Geometry: final body of the model. Coordinates: model frame, mm. A direction names the side the tool comes from. Give positions to 0.01 mm unless a question says otherwise; leave off trailing zeros. Order: outer loops, then holes, each group sorted by start corner. A loop starts at its lowest first (then second) coordinate and runs counter-clockwise, first axis right, second up. Notation, with made-up numbers: (83.5, -12) - (123.5, -12) arc R26 cw to (123.5, 8) - close; hole circle Ø3 at (51.25, 27). An arc over 180 degrees is marked (long way). One line per item, written item: value.
```python
from build123d import *

# Parameters (mm, degrees)
CIRCULARBAND_W               = 50
CIRCULARBAND_H               = 2.5
BASE_REVOLVE_ANGLE           = 120
BASE_REVOLVE_OTHER_WAY_ANGLE = 120
SKETCH9_OUTSIDE_W            = 80.09
SKETCH9_OUTSIDE_H            = 108.84
HEAD1_DEPTH                  = 53.5
SKETCH10_OUTSIDE_W           = 80.09
SKETCH10_OUTSIDE_H           = 108.84
TAIL1_DEPTH                  = 53.5


with BuildPart() as part:
    # circularband → Base-Revolve (revolve)
    with BuildSketch(Plane.XY):
        with Locations((0, 51.25)):
            Rectangle(CIRCULARBAND_W, CIRCULARBAND_H)
    revolve(axis=Axis((0, 0, 0), (1, 0, 0)), revolution_arc=BASE_REVOLVE_ANGLE)

    # circularband → Base-Revolve other way (revolve)
    with BuildSketch(Plane.XY):
        with Locations((0, 51.25)):
            Rectangle(CIRCULARBAND_W, CIRCULARBAND_H)
    revolve(axis=Axis((0, 0, 0), (-1, 0, 0)), revolution_arc=BASE_REVOLVE_OTHER_WAY_ANGLE)

    # Sketch9 outside → head1 (cut, through all)
    with BuildSketch(Plane.XY):
        with Locations((0, 13.125)):
            Rectangle(SKETCH9_OUTSIDE_W, SKETCH9_OUTSIDE_H)
        Polygon((-11.25, 52.5), (11.25, 52.5), (11.25, 19.301270189), (25, 19.301270189), (0, -24), (-25, 19.301270189), (-11.25, 19.301270189), align=None, mode=Mode.SUBTRACT)
    extrude(amount=-HEAD1_DEPTH, mode=Mode.SUBTRACT)

    # Sketch10 outside → tail1 (cut, through all)
    with BuildSketch(Plane.XY):
        with Locations((0, 13.125)):
            Rectangle(SKETCH10_OUTSIDE_W, SKETCH10_OUTSIDE_H)
        Polygon((0, -6.764428415), (11.25, -26.25), (11.25, 52.5), (-11.25, 52.5), (-11.25, -26.25), align=None, mode=Mode.SUBTRACT)
    extrude(amount=TAIL1_DEPTH, mode=Mode.SUBTRACT)


solid = part.part
```
1) First-contact query: pin 1 (1.5 mm diameter, centred on x = 8.5, y = 29, fed in from -Z); pin 2 (0.8 mm diameter, centred on x = 15.5, z = -48, fed in from +Y); pin 3 (3 mm diameter, centred on x = 18, y = 20, fed in from -Z). Flat tips, straight axial feed; report the tip coordinate or a pass-through.
Answers below:
pin 1: z = -44.25
pin 2: y = 19.3
pin 3: z = -49.13
2) Section A-A, the plane y = 8. Return loops of the section in (x, z), then the cut area to 3 significant figures.
Answers below:
outline: (-18.48, -51.89) - (18.48, -51.89) - (18.48, -49.36) - (-18.48, -49.36) - close; (-11.25, 49.36) - (11.25, 49.36) - (11.25, 51.89) - (-11.25, 51.89) - close
area: 150 mm^2
3) Mould query, pull axis Z, two halves, no side actions, for faces 4 (the face through (0.35, 52.425, 2.802)), 5 (the face through (0.35, 45.61, -20.49)), 6 (the face through (18, 19.301, -47)). Classes: released by +Z, released by -Z, zero draft, split by the parting line, or undercut.
Answers below:
face 4: split by the parting line
face 5: undercut
face 6: zero draft
4) Section C-C, the plane z = 0. Return loops of the section in (x, y).
Answers below:
outline: (-11.25, 50) - (11.25, 50) - (11.25, 52.5) - (-11.25, 52.5) - close
5) Material intervals for line 1 along Z through (x, y) = (-1, 0); line 2 along Y through (x, z) = (-4, 0); line 3 along Z through (x, y) = (2.5, 6), sorted ascending.
Answers below:
line 1: -52.5 to -50, 50 to 52.5
line 2: 50 to 52.5
line 3: -52.16 to -49.64, 49.64 to 52.16
6) Section B-B, the plane y = -9. Return loops of the section in (x, z), then the cut area to 3 significant figures.
Answers below:
outline: (-11.25, 49.18) - (-1.29, 49.18) - (-1.29, 51.72) - (-11.25, 51.72) - close; (-8.66, -51.72) - (8.66, -51.72) - (8.66, -49.18) - (-8.66, -49.18) - close; (1.29, 49.18) - (11.25, 49.18) - (11.25, 51.72) - (1.29, 51.72) - close
area: 94.6 mm^2
7) Set-up query: faces 1 (the face through (12.558, -2.248, -50.721)), 2 (the face through (-18, 19.301, -47)), 3 (the face through (-12.44, -2.45, -50.4)). Return all of +Z, -Z, +X, -X, +Y, -Y with unobstructed straight access to the full face (end or side cutting, diameter ignored); none if empty.
Answers below:
face 1: -Z, +X, -Y
face 2: +Z, -Z, -X, +Y
face 3: -Z, -X, -Y
8) Section D-D, the plane x = 2.5. Return loops of the section in (y, z), then the cut area to 3 significant figures.
Answers below:
outline: (-19.67, -48.68) arc R52.5 ccw (long way) to (-11.09, 51.31) - (-11.09, 48.75) arc R50 cw (long way) to (-19.67, -45.97) - close
area: 481 mm^2
